Can you work these out from the drawing? Everything is in mm from the part's minimum corner. Coordinates: 2 decimals unless noted, no trailing zeros. Order: outer loops, then holes, each group sorted by start corner. A loop starts at its lowest first (then second) coordinate and runs counter-clockwise, first axis right, second up. Notation, with made-up numbers: (89, 58.25) - (105, 58.25) arc R13 cw to (105, 72.25) - close; hole circle Ø5 at (14, 20). An arc over 180 degrees is marked (long way). One line per item, written item: value.
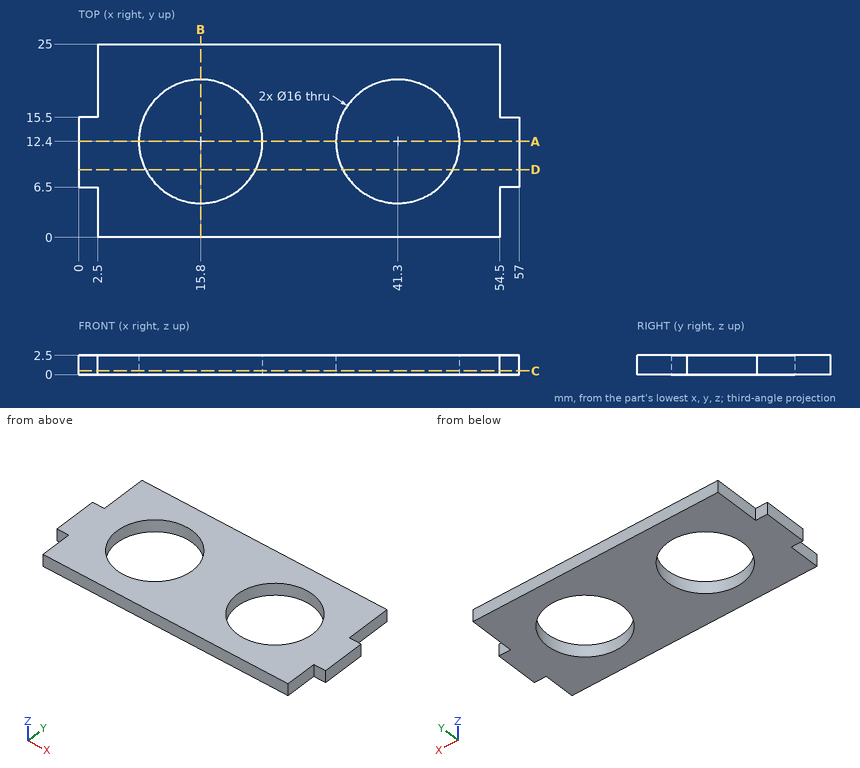
Item 1: I'm going to push flat-ended pins straight in: pin 1 Ø0.8 at (y, z) = (20, 1) entering from -X; pin 2 Ø0.8 at (x, z) = (0.5, 1) entering from -Y; pin 3 Ø0.8 at (y, z) = (2.5, 1.5) entering from +X. Where does each tip first touch, or does it pass through?
Conclusion:
pin 1: x = 2.5
pin 2: y = 6.5
pin 3: x = 54.5
Item 2: I want a section at B-B on x = 15.8. Please give me the cut outline in (y, z).
Conclusion:
outline: (0, 0) - (4.4, 0) - (4.4, 2.5) - (0, 2.5) - close; (20.4, 0) - (25, 0) - (25, 2.5) - (20.4, 2.5) - close
Item 3: I want a section at A-A on y = 12.4. Please give me the cut outline in (x, z).
Conclusion:
outline: (0, 0) - (7.8, 0) - (7.8, 2.5) - (0, 2.5) - close; (23.8, 0) - (33.3, 0) - (33.3, 2.5) - (23.8, 2.5) - close; (49.3, 0) - (57, 0) - (57, 2.5) - (49.3, 2.5) - close
Item 4: I want a section at C-C on z = 0.5. Please give me the cut outline in (x, y).
Conclusion:
outline: (0, 6.5) - (2.5, 6.5) - (2.5, 0) - (54.5, 0) - (54.5, 6.5) - (57, 6.5) - (57, 15.5) - (54.5, 15.5) - (54.5, 25) - (2.5, 25) - (2.5, 15.5) - (0, 15.5) - close; hole circle Ø16 at (15.8, 12.4); hole circle Ø16 at (41.3, 12.4)
Item 5: I want a section at D-D on y = 8.75. Please give me the cut outline in (x, z), then the cut area to 3 significant figures.
Conclusion:
outline: (0, 0) - (8.68, 0) - (8.68, 2.5) - (0, 2.5) - close; (22.92, 0) - (34.18, 0) - (34.18, 2.5) - (22.92, 2.5) - close; (48.42, 0) - (57, 0) - (57, 2.5) - (48.42, 2.5) - close
area: 71.3 mm²
Item 6: If I drill on probe 1 along X at (y, z) = (19.75, 0.8); probe 2 along X at (y, z) = (14, 1.95); probe 3 along Y at (x, z) = (41.3, 1.85), over which ranges is the centre line in solid material (lowest first)?
Conclusion:
probe 1: 2.5 to 12.64, 18.96 to 38.14, 44.46 to 54.5
probe 2: 0 to 7.96, 23.64 to 33.46, 49.14 to 57
probe 3: 0 to 4.4, 20.4 to 25
